```python
from build123d import *

# Parameters (mm, degrees)
SKETCH1_W                           = 44.45
SKETCH1_H                           = 50.8
BOSS_EXTRUDE1_DEPTH                 = 3.175
BOSS_EXTRUDE2_DEPTH                 = 3.175
SKETCH3_W                           = 9.525
SKETCH3_H                           = 9.525
BOSS_EXTRUDE3_DEPTH                 = 9.525
SKETCH4_R                           = 8.7376
CUT_EXTRUDE1_DEPTH                  = 7.35
F_6_32_TAPPED_HOLE1_D               = 2.7051
F_6_32_TAPPED_HOLE1_DEPTH           = 9.525
F_6_32_TAPPED_HOLE1_ON_FACE_2_D     = 2.7051
F_6_32_TAPPED_HOLE1_ON_FACE_2_DEPTH = 9.525
F_6_32_TAPPED_HOLE1_ON_FACE_3_D     = 2.7051
F_6_32_TAPPED_HOLE1_ON_FACE_3_DEPTH = 9.525


with BuildPart() as part:
    # Sketch1 → Boss-Extrude1 (new body)
    with BuildSketch(Plane.XY):
        Rectangle(SKETCH1_W, SKETCH1_H)
    extrude(amount=BOSS_EXTRUDE1_DEPTH)

    # Sketch2 → Boss-Extrude2 (add)
    with BuildSketch(Plane.XY.offset(3.175)):
        with BuildLine():
            Line((-12.7, -10.16), (-12.7, -25.4))
            Line((-12.7, -25.4), (12.7, -25.4))
            Line((12.7, -25.4), (12.7, -10.16))
            ThreePointArc((12.7, -10.16), (0, 2.54), (-12.7, -10.16))
        make_face()
    extrude(amount=BOSS_EXTRUDE2_DEPTH)

    # Sketch3 → Boss-Extrude3 (add)
    with BuildSketch(Plane.XY.offset(3.175)):
        with Locations((-17.4625, -20.6375)):
            Rectangle(SKETCH3_W, SKETCH3_H)
        with Locations((17.4625, -20.6375)):
            Rectangle(SKETCH3_W, SKETCH3_H)
    extrude(amount=BOSS_EXTRUDE3_DEPTH)

    # Sketch4 → Cut-Extrude1 (cut, through all)
    with BuildSketch(Plane.XY.offset(6.35)):
        with Locations((0, -10.16)):
            Circle(SKETCH4_R)
    extrude(amount=-CUT_EXTRUDE1_DEPTH, mode=Mode.SUBTRACT)

    # #6-32 Tapped Hole1
    with Locations(Plane(origin=(22.225, -20.6375, 7.9375), x_dir=(0, 1, 0), z_dir=(1, 0, 0))):
        with Locations((0, 0)):
            Hole(F_6_32_TAPPED_HOLE1_D / 2, depth=F_6_32_TAPPED_HOLE1_DEPTH)

    # #6-32 Tapped Hole1 on face 2
    with Locations(Plane(origin=(-22.225, -20.6375, 7.9375), x_dir=(0, 0, -1), z_dir=(-1, 0, 0))):
        with Locations((0, 0)):
            Hole(F_6_32_TAPPED_HOLE1_ON_FACE_2_D / 2, depth=F_6_32_TAPPED_HOLE1_ON_FACE_2_DEPTH)

    # #6-32 Tapped Hole1 on face 3
    with Locations(Plane(origin=(0, 21.59, 3.175), x_dir=(1, 0, 0), z_dir=(0, 0, 1))):
        with Locations((0, 0)):
            Hole(F_6_32_TAPPED_HOLE1_ON_FACE_3_D / 2, depth=F_6_32_TAPPED_HOLE1_ON_FACE_3_DEPTH)


solid = part.part
```
Geometry check sheet. Reference: the model listing, model coordinates, mm. A direction names the side the tool comes from. Give positions to 0.01 mm unless a question says otherwise; leave off trailing zeros. Write each loop counter-clockwise with the first axis right and the second up, starting at its lowest first coordinate (ties: lowest second). Pieces come first, ordered by that corner, then holes.
1) Section check C-C, the plane x = 0. Record the boundary of the cut face in (y, z) (3 decimals).
2) Release check for a two-part mould opening along X. For faces 4 (the cylindrical face through (17.4, -21.93, 8.34)), 5 (the cylindrical face through (0.279, 2.537, 4.74)), 6 (the flat face through (-12.7, -20.7, 9.5)) record: pulls with the +X half, pulls with the -X half, needs draft (parallel to the pull), parting line crosses it, or undercut.
3) Material ranges on L1, parallel to Y at x = 0, z = 1.5; L2, parallel to Y at x = 0, z = 4.5; L3, parallel to X at y = -19, z = 8 (3 decimals), recorded low to high.
4) Gauge pin test, flat ends, axial feed: pin 1 (14 mm diameter, centred on x = 0, y = -10.16, fed in from +Z); pin 2 (1 mm diameter, centred on y = -13, z = 5, fed in from -X); pin 3 (5 mm diameter, centred on x = -5.5, z = 8.5, fed in from +Y); pin 4 (7.5 mm diameter, centred on x = 19, z = 7.5, fed in from +Y) (3 decimals). Record the tip position at first contact, or that the pin passes through.
5) Section check D-D, the plane z = 1. Record the boundary of the cut face in (x, y) (3 decimals).
6) Access from +Z, -Z, +X, -X, +Y, -Y to the whole of each face (thin tool, end or side, straight path). Record for faces 1 (the flat face through (0, 10, 3.175)), 2 (the flat face through (-6, -17, 6.35)), 3 (the flat face through (12.7, -13, 5)).
7) Section check A-A, the plane z = 5.25. Record the boundary of the cut face in (x, y) (3 decimals).
8) Section check B-B, the plane y = 21.59. Record the boundary of the cut face in (x, z) (3 decimals), and give its area (3 significant figures).
Computed:
1. outline: (-25.4, 0) - (-18.898, 0) - (-18.898, 6.35) - (-25.4, 6.35) - close; (-1.422, 0) - (20.237, 0) - (20.237, 3.175) - (2.54, 3.175) - (2.54, 6.35) - (-1.422, 6.35) - close; (22.943, 0) - (25.4, 0) - (25.4, 3.175) - (22.943, 3.175) - close
2. face 4: needs draft
2. face 5: parting line crosses it
2. face 6: undercut
3. L1: y = -25.4 to -18.9, -1.42 to 20.24, 22.94 to 25.4
3. L2: y = -25.4 to -18.9, -1.42 to 2.54
3. L3: x = -22.225 to -12.7, 12.7 to 22.225
4. pin 1: passes through
4. pin 2: stops at x = -12.7
4. pin 3: stops at y = 1.82
4. pin 4: stops at y = -15.875
5. outline: (-22.225, -25.4) - (22.225, -25.4) - (22.225, 25.4) - (-22.225, 25.4) - close; hole circle Ø17.475 at (0, -10.16); hole circle Ø2.705 at (0, 21.59)
6. face 1: +Z, +Y
6. face 2: +Z, +Y, -Y
6. face 3: +Z, +X, +Y
7. outline: (-22.225, -25.4) - (22.225, -25.4) - (22.225, -15.875) - (12.7, -15.875) - (12.7, -10.16) arc R12.7 ccw to (-12.7, -10.16) - (-12.7, -15.875) - (-22.225, -15.875) - close; hole circle Ø17.475 at (0, -10.16)
8. outline: (-22.225, 0) - (-1.353, 0) - (-1.353, 3.175) - (-22.225, 3.175) - close; (1.353, 0) - (22.225, 0) - (22.225, 3.175) - (1.353, 3.175) - close
8. area: 133 mm2
